```python
from build123d import *

# Parameters (mm, degrees)
SKETCH1_W           = 38
SKETCH1_H           = 23
BOSS_EXTRUDE1_DEPTH = 18
SKETCH3_R           = 0.4
BOSS_EXTRUDE3_DEPTH = 5
SKETCH4_R           = 0.4
BOSS_EXTRUDE4_DEPTH = 5
SKETCH5_R           = 0.4
BOSS_EXTRUDE5_DEPTH = 5
SKETCH6_R           = 0.4
BOSS_EXTRUDE6_DEPTH = 5


with BuildPart() as part:
    # Sketch1 → Boss-Extrude1 (new body)
    with BuildSketch(Plane.XZ):
        with Locations((0, -0.939824945)):
            Rectangle(SKETCH1_W, SKETCH1_H)
    extrude(amount=-BOSS_EXTRUDE1_DEPTH)

    # Sketch3 → Boss-Extrude3 (add)
    with BuildSketch(Plane.XZ):
        with Locations(Location((16.8, -9.939824945, 0), (0, 0, 270))):
            Circle(SKETCH3_R)
    extrude(amount=BOSS_EXTRUDE3_DEPTH)

    # Sketch4 → Boss-Extrude4 (add)
    with BuildSketch(Plane.XZ):
        with Locations(Location((-16.8, -3.939824945, 0), (0, 0, 270))):
            Circle(SKETCH4_R)
    extrude(amount=BOSS_EXTRUDE4_DEPTH)

    # Sketch5 → Boss-Extrude5 (add)
    with BuildSketch(Plane.XZ):
        with Locations(Location((16.8, 8.060175055, 0), (0, 0, 270))):
            Circle(SKETCH5_R)
    extrude(amount=BOSS_EXTRUDE5_DEPTH)

    # Sketch6 → Boss-Extrude6 (add)
    with BuildSketch(Plane.XZ):
        with Locations(Location((-16.8, 2.060175055, 0), (0, 0, 270))):
            Circle(SKETCH6_R)
    extrude(amount=BOSS_EXTRUDE6_DEPTH)


solid = part.part
```
Check sheet for the modelled part. Datum: model origin and axes. Units: mm. A direction names the side the tool comes from. Coordinates: 2 decimals unless noted, no trailing zeros. Write each loop counter-clockwise with the first axis right and the second up, starting at its lowest first coordinate (ties: lowest second). Pieces come first, ordered by that corner, then holes. Notation, with made-up numbers: M 45,14.5 L 101,14.5 A22 ccw 101,22.5 Z; hole C 11.5,25 d5. An arc over 180 degrees is marked long. Use one line per item in the form item = value.
Item 1: Gauge pin test, flat end, axial feed: pin 1 Ø10 at (x, z) = (-7.5, -6.5) entering from -Y. Record the tip position at first contact, or that the pin passes through.
Answer below:
pin_1 = 0
Item 2: Set-up check for faces 1 (the face through (17.14, -2.46, 7.85)), 2 (the face through (0, 9, -12.44)): record each of +Z, -Z, +X, -X, +Y, -Y from which the full face is reachable in a straight line by a thin tool's end or side.
Answer below:
face_1 = -Y
face_2 = -Z, +X, -X, +Y, -Y
Item 3: Sectioned sample at C-C, the plane x = 2.5. Record the cut outline in (y, z).
Answer below:
outline = M 0,-12.44 L 18,-12.44 L 18,10.56 L 0,10.56 Z
Item 4: Sectioned sample at A-A, the plane y = -1. Record the cut outline in (x, z).
Answer below:
outline = C -16.8,-3.94 d0.8; C -16.8,2.06 d0.8; C 16.8,-9.94 d0.8; C 16.8,8.06 d0.8
Item 5: Material ranges on L1, parallel to Y at x = -8.5, z = 7.75; L2, parallel to X at y = -2.25, z = 8, recorded low to high. Write a range as from..to.
Answer below:
L1 = 0..18
L2 = 16.4..17.2
Item 6: Sectioned sample at B-B, the plane z = -5. Record the cut outline in (x, y).
Answer below:
outline = M -19,0 L 19,0 L 19,18 L -19,18 Z
